Design review of the part built by this model. Coordinates are the model's own, in mm. Face numbers are marked on the shaded views. Coordinates: 2 decimals unless noted, no trailing zeros. Loops run counter-clockwise (first coordinate to the right, second up) from the corner with the lowest first, then second, coordinate; pieces in that order, holes last. Notation, with made-up numbers: (82.5, 66.5) - (86.5, 66.5) arc R26 ccw to (86.5, 97.5) - close; hole circle Ø8 at (56, 36). An arc over 180 degrees is marked (long way). Use one line per item in the form item = value. Start each with the question number.
(1) For L1, parallel to Y at x = 0, z = 3; L2, parallel to Y at x = 0, z = 20.5; L3, parallel to Z at x = 4, y = 8, list the stretches that pass through material, from the lowest coordinate up.
(2) Clearance check with flat-ended pins moving along their axes: pin 1 Ø3 at (y, z) = (-2.5, 5) entering from +X; pin 2 Ø1 at (x, z) = (-10, 28) entering from +Y; pin 3 Ø10 at (x, z) = (1.5, 16.5) entering from +Y. State where each tip first meets the part, or that it passes through.
(3) The part is to be moulded in two halves that separate along X. For the marked faces 1, 2 and 3, say which applies: pulls with the +X half, pulls with the -X half, needs draft (parallel to the pull), parting line crosses it, or undercut.
(4) Add section C-C (z = 3.5). State the section outline as (x, y) points.
(5) Add section A-A (x = 20). State the section outline as (y, z) points, plus the area to 3 significant figures.
(6) Add section D-D (y = -6). State the section outline as (x, z) points, plus the area to 3 significant figures.
```python
from build123d import *

# Parameters (mm, degrees)
ESQUISSE1_R                             = 25
BOSS_EXTRU_1_DEPTH                      = 5
ESQUISSE2_R                             = 13
ESQUISSE2_R_2                           = 10.25
BOSS_EXTRU_2_DEPTH                      = 30
ESQUISSE3_R                             = 1.5
ENL_V_MAT_EXTRU_1_DEPTH                 = 47.368092477
R_P_TITION_CIRCULAIRE1_COUNT            = 4
DIAM_TRE_DU_PER_AGE_3_0_3_1_D           = 3
DIAM_TRE_DU_PER_AGE_3_0_3_1_ON_FACE_2_D = 3


with BuildPart() as part:
    # Esquisse1 → Boss.-Extru.1 (new body)
    with BuildSketch(Plane.XY):
        Circle(ESQUISSE1_R)
    extrude(amount=BOSS_EXTRU_1_DEPTH)

    # Esquisse2 → Boss.-Extru.2 (add)
    with BuildSketch(Plane.XY.offset(5)):
        Circle(ESQUISSE2_R)
        Circle(ESQUISSE2_R_2, mode=Mode.SUBTRACT)
    extrude(amount=BOSS_EXTRU_2_DEPTH)

    # Esquisse3 → Enlèv. mat.-Extru.1 (cut, through all)
    with BuildSketch(Plane.XY.offset(5)):
        with Locations((0, 20)):
            Circle(ESQUISSE3_R)
    enl_v_mat_extru_1 = extrude(amount=-ENL_V_MAT_EXTRU_1_DEPTH, mode=Mode.SUBTRACT)

    # Répétition circulaire1: Enlèv. mat.-Extru.1 ×4 about axis
    r_p_tition_circulaire1_axis = Axis((0, 0, 0), (0, 0, 1))
    for i in range(1, R_P_TITION_CIRCULAIRE1_COUNT):
        add(enl_v_mat_extru_1.rotate(r_p_tition_circulaire1_axis, i * 360 / R_P_TITION_CIRCULAIRE1_COUNT), mode=Mode.SUBTRACT)

    # Diamètre du perçage Ø3.0 (3)1 (through all)
    with Locations(Plane(origin=(-0.03314831, -12.999957738, 25), x_dir=(-0.999996749076, 0.002549870024, 0), z_dir=(-0.002549870024, -0.999996749076, 0))):
        with Locations((0, 0)):
            Hole(DIAM_TRE_DU_PER_AGE_3_0_3_1_D / 2)

    # Diamètre du perçage Ø3.0 (3)1 on face 2 (through all)
    with Locations(Plane(origin=(-12.999956307, 0.03370475, 15), x_dir=(-0.002592999062, -0.999996638172, 0), z_dir=(-0.999996638172, 0.002592999062, 0))):
        with Locations((0, 0)):
            Hole(DIAM_TRE_DU_PER_AGE_3_0_3_1_ON_FACE_2_D / 2)


solid = part.part
```
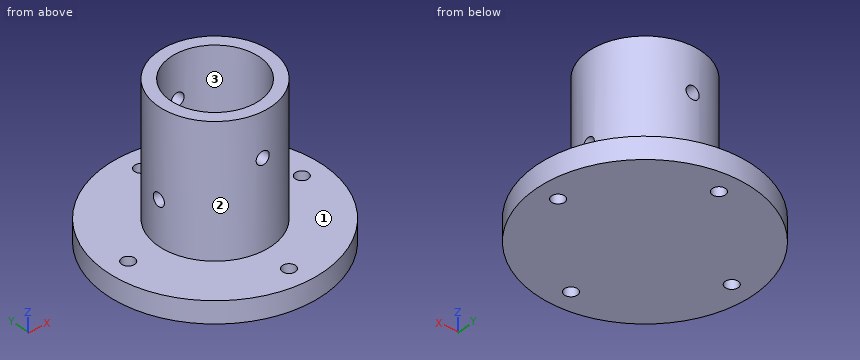
Computed values:
q1.L1 = -25 to -21.5, -18.5 to 18.5, 21.5 to 25
q1.L2 = -13 to -10.25, 10.25 to 13
q1.L3 = 0 to 5
q2.pin_1 = 24.98
q2.pin_2 = 8.87
q2.pin_3 = 13
q3.face_1 = needs draft
q3.face_2 = parting line crosses it
q3.face_3 = undercut
q4.outline = circle Ø50 at (0, 0); hole circle Ø3 at (-20, 0); hole circle Ø3 at (0, -20); hole circle Ø3 at (0, 20); hole circle Ø3 at (20, 0)
q5.outline = (-15, 0) - (-1.5, 0) - (-1.5, 5) - (-15, 5) - close; (1.5, 0) - (15, 0) - (15, 5) - (1.5, 5) - close
q5.area = 135 mm^2
q6.outline = (-24.27, 0) - (24.27, 0) - (24.27, 5) - (11.53, 5) - (11.53, 35) - (8.31, 35) - (8.31, 5) - (-8.31, 5) - (-8.31, 35) - (-11.53, 35) - (-11.53, 5) - (-24.27, 5) - close
q6.area = 436 mm^2
